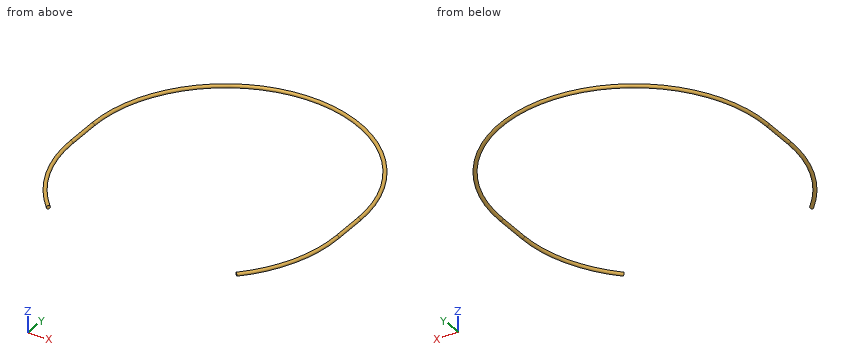
```python
from build123d import *

# Parameters (mm, degrees)
SWEEP1_PROFILE_R = 2.5


with BuildPart() as part:
    # Sweep1: sweep along a path in Sketch10
    with BuildLine(Plane.XY) as sweep1_path:
        ThreePointArc((-137.885822331, -185.885822331), (-180.15650884, -122.623269311), (-195, -48))
        Line((-195, -48), (-195, 0))
        ThreePointArc((-195, 0), (0, 195), (195, 0))
        Line((195, 0), (195, -48))
        ThreePointArc((195, -48), (180.15650884, -122.623269311), (137.885822331, -185.885822331))
    # Sweep1 profile (on start of the path) → Sweep1 (sweep)
    with BuildSketch(Plane(origin=(-137.885822331, -185.885822331, 0), x_dir=(0.7071067811865517, 0.7071067811865435, 0), z_dir=(-0.7071067811865435, 0.7071067811865517, 0))):
        Circle(SWEEP1_PROFILE_R)
    sweep(path=sweep1_path.line)


solid = part.part
```
CAD build for the part. Positions are in the model's coordinates, mm. Give positions to 0.01 mm unless a question says otherwise; leave off trailing zeros. Write each loop counter-clockwise with the first axis right and the second up, starting at its lowest first coordinate (ties: lowest second). Pieces come first, ordered by that corner, then holes. Notation, with made-up numbers: M -35,51 L -3,51 A23 cw -3,88 Z; hole C 56.25,13.5 d10. An arc over 180 degrees is marked long. Return JSON: item names as keys, results as strings. Group by question number.
(1) Band-saw the part on A-A (z = 0.95). Give the cut face in (x, y).
(2) Flat gauge pins, fed straight in: pin 1 Ø1 at (y, z) = (28.5, -1.5) entering from -X; pin 2 Ø1 at (x, z) = (10, -1) entering from -Y. Where does each tip first touch, or does it go through?
(3) Drill centre lines: L1, parallel to X at y = -34.5, z = -0.55; L2, parallel to Y at x = -151.5, z = 1.1; L3, parallel to X at y = -46, z = 1.1 (3 decimals). Where is each one in solid material? Low to high. Write a range as [from, to].
Entries:
{
 "1": {"outline": "M -197.31,-48 A197.31 ccw -139.52,-187.52 L -136.25,-184.25 A192.69 cw -192.69,-48 L -192.69,0 A192.69 cw 192.69,0 L 192.69,-48 A192.69 cw 136.25,-184.25 L 139.52,-187.52 A197.31 ccw 197.31,-48 L 197.31,0 A197.31 ccw -197.31,0 Z"},
 "2": {"pin 1": "stops at x = -195.23", "pin 2": "stops at y = 192.29"},
 "3": {"L1": "x = [-197.44, -192.56], [192.56, 197.44]", "L2": "y = [-174.31, -167.17], [119.17, 126.31]", "L3": "x = [-197.245, -192.755], [192.755, 197.245]"}
}
